Autodesk Inventor part; units mm, degrees
ref_plane "YZ Plane" through (0, 0, 0) normal (1, 0, 0) x (0, 1, 0)
ref_plane "XZ Plane" through (0, 0, 0) normal (0, 1, 0) x (-1, 0, 0)
ref_plane "XY Plane" through (0, 0, 0) normal (0, 0, 1) x (1, 0, 0)
sketch "Sketch1" plane through (0, 0, 0) normal (1, 0, 0) x (0, 1, 0)
  line L0 (0, 0) -> (101.6, 0)
  line L1 (101.6, 0) -> (101.6, -152.4)
  line L2 (101.6, -152.4) -> (0, -152.4)
  line L3 (0, -152.4) -> (0, 0)
  circle A0 centre (50.8, -28.575) radius 14.2875
  circle A1 centre (50.8, -60.325) radius 6.35
  circle A2 centre (50.8, -92.075) radius 6.35
  circle A3 centre (50.8, -123.825) radius 14.2875
  line L4 (50.8, -28.575) -> (50.8, -123.825) construction
  circle A4 centre (88.9, -12.7) radius 3.175
  circle A5 centre (88.9, -38.1) radius 3.175
  circle A6 centre (88.9, -63.5) radius 3.175
  circle A7 centre (88.9, -88.9) radius 3.175
  circle A8 centre (88.9, -114.3) radius 3.175
  circle A9 centre (88.9, -139.7) radius 3.175
  circle A10 centre (12.7, -12.7) radius 3.175
  circle A11 centre (12.7, -38.1) radius 3.175
  circle A12 centre (12.7, -63.5) radius 3.175
  circle A13 centre (12.7, -88.9) radius 3.175
  circle A14 centre (12.7, -114.3) radius 3.175
  circle A15 centre (12.7, -139.7) radius 3.175
  point P0 (101.6, -76.2)
  point P1 (50.8, -76.2)
  point P2 (50.8, -152.4)
  dimension "d0" = 101.6
  dimension "d1" = 152.4
  dimension "d2" = 28.575
  dimension "d3" = 12.7
  dimension "d4" = 12.7
  dimension "d5" = 28.575
  dimension "d6" = 31.75
  dimension "d7" = 31.75
  dimension "d8" = 31.75
  dimension "d9" = 6.35
  dimension "d10" = 12.7
  dimension "d11" = 12.7
  dimension "d14" = 25.4
  dimension "d17" = 76.2
extrude "Extrusion1" add sketch "Sketch1" along normal blind 3.175
equation "\"d7\" = d6"
equation "\"d8\" = d7"
properties part number "CH-1-02-RearGearboxHousingMotorSide"
Can you work these out from the model? Positions are in its coordinate system, mm. Coordinates: 2 decimals unless noted, no trailing zeros. Order: outer loops, then holes, each group sorted by start corner. A loop starts at its lowest first (then second) coordinate and runs counter-clockwise, first axis right, second up. Notation, with made-up numbers: M 22.5,4.25 L 74.5,4.25 A21 ccw 74.5,22.25 Z; hole C 18,-16 d2. An arc over 180 degrees is marked long. Answer as CSV lines item,"result".
(1) If we mould it in two halves opening along Z, with no side actions, what happens to faces 1 (the flat face through (0, 50, -75)), 2 (the flat face through (2, 52, -152.4)), 3 (the cylindrical face through (1.57, 12.01, -111.2))? For each: released by +Z, released by -Z, zero draft, split by the parting line, or undercut.
Geometry check:
face 1,"zero draft"
face 2,"released by -Z"
face 3,"undercut"
(2) Suppose I cut it at D-D on z = -114.3. Please give me the cut outline in (x, y) (3 decimals).
Geometry check:
outline,"M 0,0 L 3.175,0 L 3.175,9.525 L 0,9.525 Z; M 0,15.875 L 3.175,15.875 L 3.175,40.151 L 0,40.151 Z; M 0,61.449 L 3.175,61.449 L 3.175,85.725 L 0,85.725 Z; M 0,92.075 L 3.175,92.075 L 3.175,101.6 L 0,101.6 Z"
(3) Suppose I cut it at B-B on y = 12.7. Please give me the cut outline in (x, z) (3 decimals).
Geometry check:
outline,"M 0,-152.4 L 3.175,-152.4 L 3.175,-142.875 L 0,-142.875 Z; M 0,-136.525 L 3.175,-136.525 L 3.175,-117.475 L 0,-117.475 Z; M 0,-111.125 L 3.175,-111.125 L 3.175,-92.075 L 0,-92.075 Z; M 0,-85.725 L 3.175,-85.725 L 3.175,-66.675 L 0,-66.675 Z; M 0,-60.325 L 3.175,-60.325 L 3.175,-41.275 L 0,-41.275 Z; M 0,-34.925 L 3.175,-34.925 L 3.175,-15.875 L 0,-15.875 Z; M 0,-9.525 L 3.175,-9.525 L 3.175,0 L 0,0 Z"
(4) Please list where these lines run through material, in increasing order: L1, parallel to Z at x = 1, y = 50.8 (1 decimal); L2, parallel to Y at x = 0.6, z = -87; L3, parallel to Y at x = 1.25, z = -88.5.
Geometry check:
L1,"-152.4 to -138.1, -109.5 to -98.4, -85.7 to -66.7, -54 to -42.9, -14.3 to 0"
L2,"0 to 10.16, 15.24 to 46.98, 54.62 to 86.36, 91.44 to 101.6"
L3,"0 to 9.55, 15.85 to 45.55, 56.05 to 85.75, 92.05 to 101.6"
(5) Suppose I cut it at C-C on y = 59. Please give me the cut outline in (x, z) (3 decimals), plus the area to 3 significant figures.
Geometry check:
outline,"M 0,-152.4 L 3.175,-152.4 L 3.175,-135.525 L 0,-135.525 Z; M 0,-112.125 L 3.175,-112.125 L 3.175,-40.275 L 0,-40.275 Z; M 0,-16.875 L 3.175,-16.875 L 3.175,0 L 0,0 Z"
area,"335 mm^2"
(6) Suppose I cut it at A-A on z = -12.7. Please give me the cut outline in (x, y) (3 decimals), plus the area to 3 significant figures.
Geometry check:
outline,"M 0,0 L 3.175,0 L 3.175,9.525 L 0,9.525 Z; M 0,15.875 L 3.175,15.875 L 3.175,85.725 L 0,85.725 Z; M 0,92.075 L 3.175,92.075 L 3.175,101.6 L 0,101.6 Z"
area,"282 mm^2"
(7) I'm going to push a flat-ended pin straight in: pin 1 (5 mm diameter, centred on y = 12.7, z = -63.5, fed in from +X). Where does the tip first touch, or does it pass through?
Geometry check:
pin 1,"through"
